Geometry check sheet. Reference: the model listing, model coordinates, mm. Face numbers are marked on the shaded views. A direction names the side the tool comes from. Coordinates: 2 decimals unless noted, no trailing zeros. Write each loop counter-clockwise with the first axis right and the second up, starting at its lowest first coordinate (ties: lowest second). Pieces come first, ordered by that corner, then holes. Notation, with made-up numbers: M 38,-31 L 78,-31 A30 ccw 78,0 Z; hole C 22,61 d1. An arc over 180 degrees is marked long. Write each question's results on one line, items separated by ' | '.
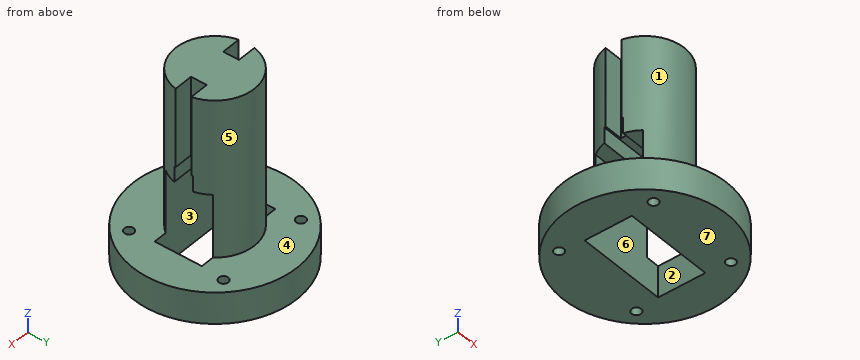
```python
from build123d import *

# Parameters (mm, degrees)
F0_W     = 12.5
F0_H     = 50
F2_W     = 8
F2_H     = 5
F3_DEPTH = 37.5
F4_W     = 28.5
F4_H     = 6
F5_DEPTH = 35
F6_W     = 28.5
F6_H     = 4.5
F7_DEPTH = 30
F6_H_2   = 15
F6_R     = 1.5
F8_DEPTH = 11


with BuildPart() as f1:
    # F0 (on Front) → F1 (revolve)
    with BuildSketch(Plane.XZ):
        with Locations((6.25, -1.05346)):
            Rectangle(F0_W, F0_H)
        Polygon((12.5, -26.05346), (0, -26.05346), (0, -36.05346), (26, -36.05346), (26, -26.05346), align=None)
    revolve(axis=Axis((0, 0, -1.05346), (0, 0, -1)))

    # F2 (on Top) → F3 (cut, symmetric)
    with BuildSketch(Plane.XY):
        with Locations((-10.25, 0)):
            Rectangle(F2_W, F2_H)
        with Locations((10.25, 0)):
            Rectangle(F2_W, F2_H)
    extrude(amount=F3_DEPTH, both=True, mode=Mode.SUBTRACT)

    # F4 (on face) → F5 (cut)
    with BuildSketch(Plane(origin=(0, 0, -36.05346), x_dir=(1, 0, 0), z_dir=(0, 0, -1))):
        Rectangle(F4_W, F4_H)
    extrude(amount=-F5_DEPTH, mode=Mode.SUBTRACT)

    # F6 (on face) → F7 (cut)
    with BuildSketch(Plane(origin=(0, 0, -36.05346), x_dir=(1, 0, 0), z_dir=(0, 0, -1))):
        with Locations((0, 5.25)):
            Rectangle(F6_W, F6_H)
        with Locations((0, -5.25)):
            Rectangle(F6_W, F6_H)
    extrude(amount=-F7_DEPTH, mode=Mode.SUBTRACT)

    # F6 (on face) → F8 (cut)
    with BuildSketch(Plane(origin=(0, 0, -36.05346), x_dir=(1, 0, 0), z_dir=(0, 0, -1))):
        Rectangle(F6_W, F6_H_2)
        with Locations((15, -15)):
            Circle(F6_R)
        with Locations((-15, -15)):
            Circle(F6_R)
        with Locations((15, 15)):
            Circle(F6_R)
        with Locations((-15, 15)):
            Circle(F6_R)
    extrude(amount=-F8_DEPTH, mode=Mode.SUBTRACT)


solid = f1.part
```
Q1. Sectioned sample at B-B on x = 0. Record the cut outline in (y, z), and give its area (3 significant figures).
Geometry check:
outline: M -26,-36.05 L -7.5,-36.05 L -7.5,-6.05 L -3,-6.05 L -3,-1.05 L 3,-1.05 L 3,-6.05 L 7.5,-6.05 L 7.5,-36.05 L 26,-36.05 L 26,-26.05 L 12.5,-26.05 L 12.5,23.95 L -12.5,23.95 L -12.5,-26.05 L -26,-26.05 Z | area: 1,290 mm2
Q2. Scan lines: probe 1 along Y at (x, z) = (-15, -29); probe 2 along Z at (x, y) = (-2, -14). Record each from-to range of solid material in increasing order.
Geometry check:
probe 1: y = -21.24 to -16.5, -13.5 to 13.5, 16.5 to 21.24 | probe 2: z = -36.05 to -26.05
Q3. Depth check by flat-ended pin: P1, Ø1.8, axis at x = -9, z = 16, coming from the +Y side; P2, Ø3, axis at x = 10, z = 8, coming from the -Y side; P3, Ø3, axis at x = 9.5, z = 7, coming from the +Y side. Enter the tip coordinate at first touch or a pass-through.
Geometry check:
P1: stops at y = 9.52 | P2: stops at y = -9.17 | P3: stops at y = 9.6
Q4. Sectioned sample at C-C on y = 5. Record the cut outline in (x, z).
Geometry check:
outline: M -25.51,-36.05 L -14.25,-36.05 L -14.25,-26.05 L -25.51,-26.05 Z; M -11.46,-6.05 L 11.46,-6.05 L 11.46,23.95 L -11.46,23.95 Z; M 14.25,-36.05 L 25.51,-36.05 L 25.51,-26.05 L 14.25,-26.05 Z
Q5. Access from +Z, -Z, +X, -X, +Y, -Y to the whole of each face (thin tool, end or side, straight path). Record for the marked faces 1, 2, 3 and 4.
Geometry check:
face 1: +Z, -Y | face 2: +Z, -Z | face 3: -Z | face 4: +Z
Q6. Mould release check, pull along X, two halves, no side actions. Record for the marked faces 5, 6 and 7: pulls with the +X half, pulls with the -X half, needs draft (parallel to the pull), parting line crosses it, or undercut.
Geometry check:
face 5: parting line crosses it | face 6: undercut | face 7: needs draft
Q7. Sectioned sample at D-D on x = -11. Record the cut outline in (y, z).
Geometry check:
outline: M -23.56,-36.05 L -7.5,-36.05 L -7.5,-26.05 L -23.56,-26.05 Z; M -5.94,-6.05 L -3,-6.05 L -3,-1.05 L -2.5,-1.05 L -2.5,23.95 L -5.94,23.95 Z; M 2.5,-1.05 L 3,-1.05 L 3,-6.05 L 5.94,-6.05 L 5.94,23.95 L 2.5,23.95 Z; M 7.5,-36.05 L 23.56,-36.05 L 23.56,-26.05 L 7.5,-26.05 Z
Q8. Sectioned sample at A-A on z = 5. Record the cut outline in (x, y).
Geometry check:
outline: M -12.25,-2.5 A12.5 ccw 12.25,-2.5 L 6.25,-2.5 L 6.25,2.5 L 12.25,2.5 A12.5 ccw -12.25,2.5 L -6.25,2.5 L -6.25,-2.5 Z
